The figure shows three views and two pictorial views of one solid part (mm, origin at its lowest corner). Answer the questions. Coordinates: 2 decimals unless noted, no trailing zeros. Write each loop counter-clockwise with the first axis right and the second up, starting at its lowest first coordinate (ties: lowest second). Pieces come first, ordered by that corner, then holes. Notation, with made-up numbers: M 43.25,45 L 87.25,45 A31 ccw 87.25,84 Z; hole C 24,16.5 d1. An arc over 180 degrees is marked long. Write item = value, one per line.
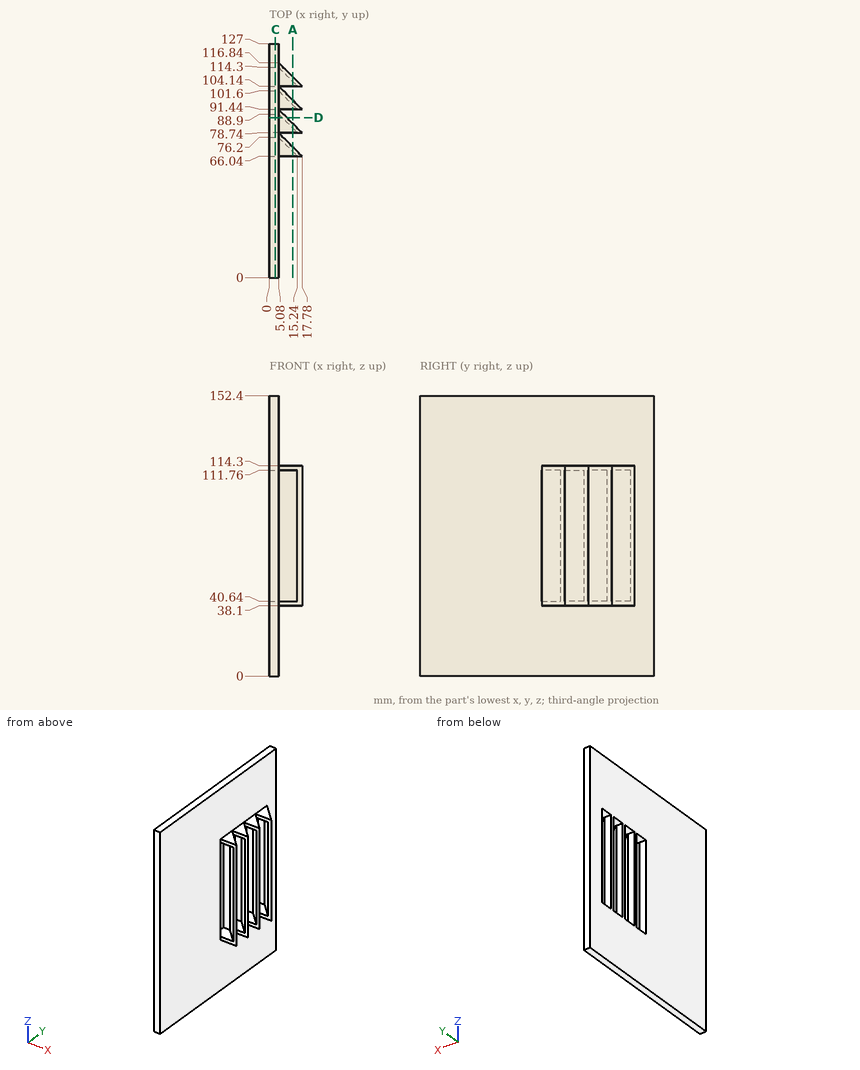
Item 1: Find section A-A (x = 12.75). State how many separate pieces and enclosed holes the cut face has, and give its area (3 significant figures).
Worked answers:
separate_pieces = 4
enclosed_holes = 0
area = 825 mm²
Item 2: Consider line 1 along Y through (x, z) = (4.75, 106); line 2 along Y through (x, z) = (11.25, 80); line 3 along Z through (x, y) = (4.25, 70). Determine where each line is inside the solid, lowest interval first. Write a range as from..to.
Worked answers:
line_1 = 0..66.04, 76.2..78.74, 88.9..91.44, 101.6..104.14, 114.3..127
line_2 = 70.03..72.57, 82.73..85.27, 95.43..97.97, 108.13..110.67
line_3 = 0..40.64, 111.76..152.4
Item 3: Find section C-C (x = 3.25). Determine the outline of the cut face in (y, z).
Worked answers:
outline = M 0,0 L 127,0 L 127,152.4 L 0,152.4 Z; hole M 66.04,40.64 L 76.2,40.64 L 76.2,111.76 L 66.04,111.76 Z; hole M 78.74,40.64 L 88.9,40.64 L 88.9,111.76 L 78.74,111.76 Z; hole M 91.44,40.64 L 101.6,40.64 L 101.6,111.76 L 91.44,111.76 Z; hole M 104.14,40.64 L 114.3,40.64 L 114.3,111.76 L 104.14,111.76 Z
Item 4: Find section D-D (y = 87). Determine the outline of the cut face in (x, z), and give its area (3 significant figures).
Worked answers:
outline = M 0,0 L 5.08,0 L 5.08,38.1 L 9.52,38.1 L 9.52,114.3 L 5.08,114.3 L 5.08,152.4 L 0,152.4 L 0,111.76 L 6.98,111.76 L 6.98,40.64 L 0,40.64 Z
area = 616 mm²
Item 5: Flat-ended cylindrical pins translate along their axes: pin 1 (1.5 mm diameter, centred on x = 6.5, y = 67, fed in from -Z); pin 2 (6 mm diameter, centred on y = 23.5, z = 132, fed in from +X); pin 3 (6.5 mm diameter, centred on x = 9, z = 84.5, fed in from -Y); pin 4 (8 mm diameter, centred on x = 10.5, y = 41.5, fed in from -Z) (3 decimals). Find the tip coordinate at first contact, or state that the pin passes through.
Worked answers:
pin_1 = 38.1
pin_2 = 5.08
pin_3 = 69.03
pin_4 = through
